```python
from build123d import *

# Parameters (mm, degrees)
SKETCH1_R           = 8
SKETCH1_R_2         = 6
BOSS_EXTRUDE1_DEPTH = 40
FILLET1_R           = 25


with BuildPart() as part:
    # Sketch1 → Boss-Extrude1 (new, symmetric)
    with BuildSketch(Plane.XY):
        Circle(SKETCH1_R)
        Circle(SKETCH1_R_2, mode=Mode.SUBTRACT)
    extrude(amount=BOSS_EXTRUDE1_DEPTH, both=True)

    # Sketch2 → Revolve1 (revolve)
    with BuildSketch(Plane(origin=(0, 0, 0), x_dir=(0, 0, -1), z_dir=(1, 0, 0)), mode=Mode.PRIVATE) as revolve1_sk:
        with BuildLine():
            Line((-25, 0), (-7.502982863, 33.73728427))
            ThreePointArc((-7.502982863, 33.73728427), (-5.661537285, 35.707899486), (-3.064404332, 36.4353241))
            Line((-3.064404332, 36.4353241), (3.064404332, 36.4353241))
            ThreePointArc((3.064404332, 36.4353241), (5.661537285, 35.707899486), (7.502982863, 33.73728427))
            Line((7.502982863, 33.73728427), (25, 0))
            Line((25, 0), (-25, 0))
        make_face()
    revolve(revolve1_sk.sketch.rotate(Axis((0, 0, -25), (0, 0, 1)), 90), axis=Axis((0, 0, -25), (0, 0, 1)))

    # Fillet1
    fillet1_edges = [part.edges().sort_by_distance(p)[0] for p in [
        (0, 8, -20.850995712),
        (0, 8, 20.850995712),
    ]]
    fillet(fillet1_edges, radius=FILLET1_R)


solid = part.part
```
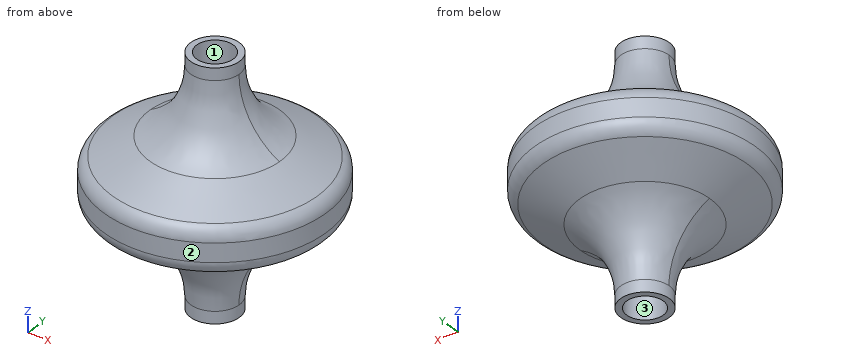
For this review, take the finished solid that the model builds, in its own axes (mm). Face numbers are marked on the shaded views. A direction names the side the tool comes from. Give positions to 0.01 mm unless a question says otherwise; leave off trailing zeros. One line per item, written item: value.
1) For P1, Ø10, axis at x = -10, z = -25, coming from the +Y side; P2, Ø10, axis at x = 26.5, z = -11, coming from the -Y side; P3, Ø9.5, axis at x = 0, y = 0, coming from the -Z side, all flat-tipped, find the tip position at first contact; note any pin that passes through.
Results are:
P1: stops at y = 11
P2: stops at y = -25.35
P3: stops at z = -25
2) For line 1 (Y direction, x = 0, z = -25.5); line 2 (Y direction, x = 0, z = -26); line 3 (X direction, y = 20, z = 2), list the stretches that pass through material, from the lowest coordinate up. Write a range as from..to.
Results are:
line 1: y = -10.33..-6, 6..10.33
line 2: y = -10.11..-6, 6..10.11
line 3: x = -30.46..30.46
3) For the marked faces 1, 2 and 3, list the 3-axis set-ups (+Z, -Z, +X, -X, +Y, -Y) from which the entire face can be reached by the end or side of a thin tool; tool diameter is ignored.
Results are:
face 1: +Z
face 2: +Z, -Z
face 3: -Z
